Source: CAD feature listing. Evaluate the final solid. Frame: model axes, mm. Round coordinates to 2 decimals unless told otherwise and drop trailing zeros. Write each loop counter-clockwise with the first axis right and the second up, starting at its lowest first coordinate (ties: lowest second). Pieces come first, ordered by that corner, then holes. Notation, with made-up numbers: (17, 57.5) -> (53, 57.5) arc R30 ccw to (53, 95.5) -> close; hole circle Ø5 at (-33, -20). An arc over 180 degrees is marked (long way). Put each result on its own line as item: value.
Autodesk Inventor part; units mm, degrees
ref_plane "YZ Plane" through (0, 0, 0) normal (1, 0, 0) x (0, 1, 0)
ref_plane "XZ Plane" through (0, 0, 0) normal (0, 1, 0) x (-1, 0, 0)
ref_plane "XY Plane" through (0, 0, 0) normal (0, 0, 1) x (1, 0, 0)
sketch "Sketch1" plane through (0, 0, 0) normal (0, 0, 1) x (1, 0, 0)
  line L0 (-750, 51.5224) -> (750, 51.5224)
  line L1 (750, 51.5224) -> (750, 0)
  line L2 (750, 0) -> (-750, 0)
  line L3 (-750, 0) -> (-750, 51.5224)
  point P0 (0, 0)
  point P1 (0, 0)
  dimension "d0" = 1500
  dimension "d1" = 51.5224
extrude "Plate1" add sketch "Sketch1" along normal blind 3
sketch "Sketch2" plane through (750, 3, 0) normal (0, -1, 0) x (1, 0, 0)
  line L0 (-1500, 0) -> (0, 0)
  line L1 (0, 0) -> (0, 30)
  line L2 (0, 30) -> (-1500, 30)
  line L3 (-1500, 30) -> (-1500, 0)
edge flange "Flange1" height 30 angle 90 thickness 3 bend radius 2.75 thickness toward (0, -1, 0) relief tear relief width 3 relief depth 1.5 edges at (0, 0, 3) wall of the first edge with corners at (-750, 3, 0) (750, 3, 0) (750, 3, 30) (-750, 3, 30)
bend "Bend1"
corner "Corner1"
sketch "Sketch5" plane through (0, 0, 0) normal (0, 0, -1) x (-1, 0, 0)
  line L0 (750, 51.5224) -> (-750, 51.5224)
  line L1 (500, 51.5224) -> (500, 31)
  line L2 (500, 31) -> (503, 31)
  line L3 (503, 31) -> (503, 51.5224)
  line L4 (750, 0) -> (-750, 0)
  point P0 (0, 0)
  dimension "d18" = 3
  dimension "d19" = 247
  dimension "d20" = 31
extrude "Extrusion1" cut sketch "Sketch5" against normal through all
pattern_linear "Rectangular Pattern1" count 3 spacing 500 along (1, 0, 0) of "Extrusion1"
sketch "Sketch6" plane through (0, 0, 0) normal (0, 0, -1) x (-1, 0, 0)
  line L0 (-750, 51.5224) -> (-750, 5.75)
  circle A0 centre (-750, 51.5224) radius 15
  line L1 (-750, 51.5224) -> (-500, 51.5224)
  point P0 (0, 0)
  point P1 (-735, 51.5224)
  point P2 (-750, 36.5224)
  dimension "d24" = 30
extrude "Extrusion2" cut sketch "Sketch6" against normal through all contours L1 A0 L0 picked at (-740.1254, 50.4098)
mirror "Mirror1" about plane through (0, 0, 0) normal (1, 0, 0) of "Extrusion2"
equation "\"d1\" = Стрингер_5"
equation "\"d18\" = Thickness"
equation "\"d2\" = Thickness"
equation "\"d3\" = BendReliefWidth"
equation "\"d4\" = BendReliefDepth"
equation "\"d5\" = MinimumRemnant"
equation "\"d6\" = TransitionRadius"
equation "\"d9\" = BendRadius"
equation "\"d10\" = CornerReliefSize"
equation "\"d11\" = GapSize"
equation "\"d12\" = JacobiRadiusSize"
equation "\"BendReliefWidth\" = Thickness"
equation "\"BendReliefDepth\" = 0.5 * Thickness"
equation "\"CornerReliefSize\" = 4 * Thickness"
equation "\"MinimumRemnant\" = 2 * Thickness"
equation "\"TransitionRadius\" = BendRadius"
equation "\"JacobiRadiusSize\" = BendRadius"
equation "\"GapSize\" = Thickness"
properties part number "МОО 055 стрингер борт 5" material "Stainless Steel"
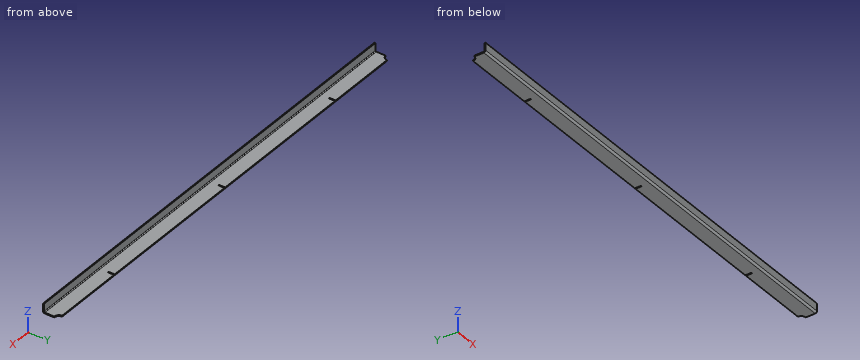
Q1. Pin query (flat end, axial travel): pin 1 (5 mm diameter, centred on x = -403, y = 15.5, fed in from +Z); pin 2 (2.5 mm diameter, centred on y = 45.5, z = 1.5, fed in from +X); pin 3 (0.9 mm diameter, centred on y = 42.5, z = 1, fed in from -X). Return the tip coordinate at first contact, or that it passes through.
Ans:
pin 1: stops at z = 3
pin 2: stops at x = 736.88
pin 3: stops at x = -738.37
Q2. Cut plane A-A on x = -199. Output: boundary loops of the cut face in (y, z), and give its area (3 significant figures).
Ans:
outline: (0, 5.75) arc R5.75 ccw to (5.75, 0) -> (51.52, 0) -> (51.52, 3) -> (5.75, 3) arc R2.75 cw to (3, 5.75) -> (3, 30) -> (0, 30) -> close
area: 230 mm^2
Q3. Cut plane B-B on z = 14.75. Output: boundary loops of the cut face in (x, y), and give its area (3 significant figures).
Ans:
outline: (-750, 0) -> (750, 0) -> (750, 3) -> (-750, 3) -> close
area: 4,500 mm^2
Q4. Material intervals for line 1 (Y direction, x = -25.5, z = 24.25); line 2 (Y direction, x = 47.5, z = 4.75), sorted ascending. Write a range as [from, to].
Ans:
line 1: y = [0, 3]
line 2: y = [0.09, 3.19]
